```python
from build123d import *

# Parameters (mm, degrees)
ESBO_O1_R                = 9.327345029
RESSALTO_EXTRUS_O1_DEPTH = 3
CORTE_EXTRUS_O1_DEPTH    = 124.439873489
FILETE1_R                = 10
ESPELHAR2_COPY_1_DEPTH   = 124.439873489


with BuildPart() as part:
    # Esboço1 → Ressalto-extrusão1 (new body)
    with BuildSketch(Plane(origin=(0, 0, 0), x_dir=(1, 0, 0), z_dir=(0, 1, 0))):
        with BuildLine():
            ThreePointArc((69.076751756, -72.307692308), (91.944752911, -39.321271752), (100, 0))
            ThreePointArc((100, 0), (91.944752911, 39.321271752), (69.076751756, 72.307692308))
            ThreePointArc((69.076751756, 72.307692308), (0, 60), (-69.076751756, 72.307692308))
            ThreePointArc((-69.076751756, 72.307692308), (-100, 0), (-69.076751756, -72.307692308))
            ThreePointArc((-69.076751756, -72.307692308), (0, -60), (69.076751756, -72.307692308))
        make_face()
        with Locations(Location((0, 0, 0), (0, 0, 270))):
            Circle(ESBO_O1_R, mode=Mode.SUBTRACT)
    extrude(amount=RESSALTO_EXTRUS_O1_DEPTH)

    # Esboço2 → Corte-extrusão1 (cut, through all)
    with BuildSketch(Plane(origin=(0, 3, 0), x_dir=(1, 0, 0), z_dir=(0, 1, 0))):
        with BuildLine():
            Line((60.350793544, 59.462439561), (78.868520735, 30.947640251))
            Line((78.868520735, 30.947640251), (85.941059495, 35.540600625))
            ThreePointArc((85.941059495, 35.540600625), (82.316182531, 43.278702541), (77.996362885, 50.651430155))
            ThreePointArc((77.996362885, 50.651430155), (73.018069946, 57.596540359), (67.423332305, 64.055399936))
            Line((67.423332305, 64.055399936), (60.350793544, 59.462439561))
        make_face()
    corte_extrus_o1 = extrude(amount=-CORTE_EXTRUS_O1_DEPTH, mode=Mode.SUBTRACT)

    # Filete1
    filete1_edges = [part.edges().sort_by_distance(p)[0] for p in [
        (-69.076751756, 1.5, -72.307692308),
        (69.076751756, 1.5, -72.307692308),
        (69.076751756, 1.5, 72.307692308),
        (-69.076751756, 1.5, 72.307692308),
    ]]
    fillet(filete1_edges, radius=FILETE1_R)

    # Espelhar1: Corte-extrusão1 across plane
    add(corte_extrus_o1.mirror(Plane(origin=(0, 0, 0), x_dir=(0, 0, 1), z_dir=(1, 0, 0))), mode=Mode.SUBTRACT)

    # Espelhar2: Corte-extrusão1 across plane
    add(corte_extrus_o1.mirror(Plane.XY), mode=Mode.SUBTRACT)

    # Espelhar2 copy 1 sketch → Espelhar2 copy 1 (cut, through all)
    with BuildSketch(Plane(origin=(0, 3, 0), x_dir=(-1, 0, 0), z_dir=(0, 1, 0))):
        with BuildLine():
            Line((60.350793544, 59.462439561), (78.868520735, 30.947640251))
            Line((78.868520735, 30.947640251), (85.941059495, 35.540600625))
            ThreePointArc((85.941059495, 35.540600625), (82.316182531, 43.278702541), (77.996362885, 50.651430155))
            ThreePointArc((77.996362885, 50.651430155), (73.018069946, 57.596540359), (67.423332305, 64.055399936))
            Line((67.423332305, 64.055399936), (60.350793544, 59.462439561))
        make_face()
    extrude(amount=-ESPELHAR2_COPY_1_DEPTH, mode=Mode.SUBTRACT)


solid = part.part
```
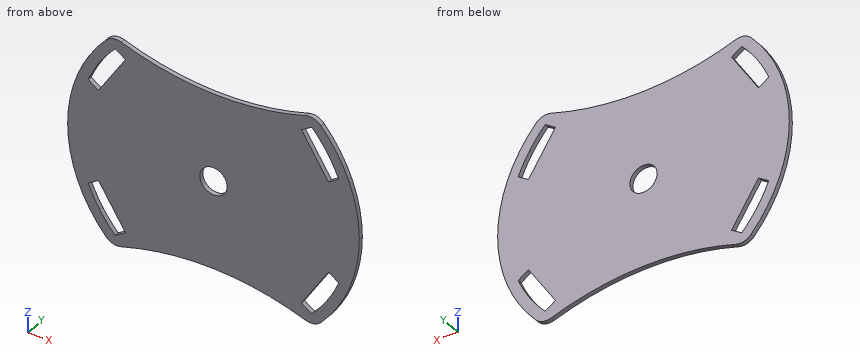
Read the model definition and answer for the solid it produces. Units are mm, in the model's axes. Give positions to 0.01 mm unless a question says otherwise; leave off trailing zeros. Write each loop counter-clockwise with the first axis right and the second up, starting at its lowest first coordinate (ties: lowest second). Pieces come first, ordered by that corner, then holes. Notation, with made-up numbers: M 69,15.25 L 87,15.25 A16 cw 87,41.25 Z; hole C 7.25,-24.75 d7. An arc over 180 degrees is marked long. Put each result on its own line as item: value. Start each with the question number.
1. Consider line 1 along X through (y, z) = (1.5, 46.5); line 2 along Z through (x, y) = (64, 1.05); line 3 along X through (y, z) = (0.75, 32.5). Determine where each line is inside the solid, lowest interval first.
2. The part is cut by section B-B, the plane z = 4. Give the vertices of the cut face in (x, y), and give its area (3 significant figures).
3. The part is cut by section A-A, the plane x = 0. Give the vertices of the cut face in (y, z).
4. The part is cut by section C-C, the plane y = 1.2. Give the number of separate pieces and of enclosed holes in the cut face, and give its area (3 significant figures).
5. Each of these flat-tipped pins is pushed along its axis until it touches: pin 1 Ø11 at (x, z) = (0, 0) entering from -Y; pin 2 Ø1 at (y, z) = (1.5, 2.5) entering from +X; pin 3 Ø1 at (y, z) = (1, -34.5) entering from +X. Where does it stop, or does it pass through?
Final values:
1. line 1: x = -88.53 to -80.54, -68.77 to 68.77, 80.54 to 88.53
1. line 2: z = -70.48 to -61.83, -53.84 to 53.84, 61.83 to 70.48
1. line 3: x = -94.57 to -81.26, -77.86 to 77.86, 81.26 to 94.57
2. outline: M -99.92,0 L -8.43,0 L -8.43,3 L -99.92,3 Z; M 8.43,0 L 99.92,0 L 99.92,3 L 8.43,3 Z
2. area: 549 mm²
3. outline: M 0,-60 L 3,-60 L 3,-9.33 L 0,-9.33 Z; M 0,9.33 L 3,9.33 L 3,60 L 0,60 Z
4. separate pieces: 1
4. enclosed holes: 5
4. area: 22,300 mm²
5. pin 1: passes through
5. pin 2: stops at x = 99.98
5. pin 3: stops at x = 94.04
